```python
from build123d import *

# Parameters (mm, degrees)
F0_W     = 152.4
F0_H     = 203.2
F0_W_2   = 101.6
F0_H_2   = 152.4
F1_DEPTH = 101.6
F2_R     = 6.35
F3_DEPTH = 25.4
F4_R     = 6.35
F5_DEPTH = 25.4


with BuildPart() as f1:
    # F0 (on Front) → F1 (new body)
    with BuildSketch(Plane.XZ):
        Rectangle(F0_W, F0_H)
        Rectangle(F0_W_2, F0_H_2, mode=Mode.SUBTRACT)
    extrude(amount=F1_DEPTH)

    # F2 (on face) → F3 (cut)
    with BuildSketch(Plane(origin=(-76.2, 0, 0), x_dir=(0, -1, 0), z_dir=(-1, 0, 0))):
        with Locations((82.55, -63.5)):
            Circle(F2_R)
        with Locations((82.55, 63.5)):
            Circle(F2_R)
    extrude(amount=-F3_DEPTH, mode=Mode.SUBTRACT)

    # F4 (on face) → F5 (cut)
    with BuildSketch(Plane.YZ.offset(76.2)):
        with Locations((-82.55, 63.5)):
            Circle(F4_R)
        with Locations((-82.55, -63.5)):
            Circle(F4_R)
    extrude(amount=-F5_DEPTH, mode=Mode.SUBTRACT)


solid = f1.part
```
The listing builds one solid part. Answer for the finished solid, in the listing's coordinates (mm). A direction names the side the tool comes from. Give positions to 0.01 mm unless a question says otherwise; leave off trailing zeros. Order: outer loops, then holes, each group sorted by start corner. A loop starts at its lowest first (then second) coordinate and runs counter-clockwise, first axis right, second up.
Item 1: Which of the six approach directions +Z, -Z, +X, -X, +Y, -Y give full straight-line access (tool end or side, diameter ignored) to faces 1 (the face through (-1, -50, -76.2)), 2 (the face through (63.68, -83.93, 57.3))?
From the geometry:
face 1: +Y, -Y
face 2: +X, -X
Item 2: The part is cut by section C-C, the plane z = 63.5. Give the vertices of the cut face in (x, y).
From the geometry:
outline: (-76.2, -101.6) - (-50.8, -101.6) - (-50.8, -88.9) - (-76.2, -88.9) - close; (-76.2, -76.2) - (-50.8, -76.2) - (-50.8, 0) - (-76.2, 0) - close; (50.8, -101.6) - (76.2, -101.6) - (76.2, -88.9) - (50.8, -88.9) - close; (50.8, -76.2) - (76.2, -76.2) - (76.2, 0) - (50.8, 0) - close
Item 3: The part is cut by section A-A, the plane y = -82.55. Give the vertices of the cut face in (x, z).
From the geometry:
outline: (-76.2, -101.6) - (76.2, -101.6) - (76.2, -69.85) - (50.8, -69.85) - (50.8, -76.2) - (-50.8, -76.2) - (-50.8, -69.85) - (-76.2, -69.85) - close; (-76.2, -57.15) - (-50.8, -57.15) - (-50.8, 57.15) - (-76.2, 57.15) - close; (-76.2, 69.85) - (-50.8, 69.85) - (-50.8, 76.2) - (50.8, 76.2) - (50.8, 69.85) - (76.2, 69.85) - (76.2, 101.6) - (-76.2, 101.6) - close; (50.8, -57.15) - (76.2, -57.15) - (76.2, 57.15) - (50.8, 57.15) - close
Item 4: The part is cut by section B-B, the plane x = -10. Give the vertices of the cut face in (y, z).
From the geometry:
outline: (-101.6, -101.6) - (0, -101.6) - (0, -76.2) - (-101.6, -76.2) - close; (-101.6, 76.2) - (0, 76.2) - (0, 101.6) - (-101.6, 101.6) - close
Item 5: Given pin 1 Ø10 at (y, z) = (-82.55, 63.5) entering from +X, flat-ended and moving along its own axis, determine where the tip first touches the part or whether it passes through.
From the geometry:
pin 1: passes through
Item 6: Find the intervals of material crossed by probe 1 along Z at (x, y) = (-68, -82); probe 2 along Z at (x, y) = (-8, -68); probe 3 along X at (y, z) = (-60, -6.5), in increasing order.
From the geometry:
probe 1: z = -101.6 to -69.83, -57.17 to 57.17, 69.83 to 101.6
probe 2: z = -101.6 to -76.2, 76.2 to 101.6
probe 3: x = -76.2 to -50.8, 50.8 to 76.2
Item 7: For a pull along Y with two mould halves and no side action, classify faces 3 (the face through (-52, 0, 1)), 4 (the face through (-63.68, -81.17, 57.3)), 5 (the face through (-50.8, -50, -1)) as pulls with the +Y half, pulls with the -Y half, needs draft (parallel to the pull), parting line crosses it, or undercut.
From the geometry:
face 3: pulls with the +Y half
face 4: undercut
face 5: needs draft
Item 8: The part is cut by section D-D, the plane z = -49. Give the vertices of the cut face in (x, y), and give its area (3 significant figures).
From the geometry:
outline: (-76.2, -101.6) - (-50.8, -101.6) - (-50.8, 0) - (-76.2, 0) - close; (50.8, -101.6) - (76.2, -101.6) - (76.2, 0) - (50.8, 0) - close
area: 5,160 mm2
